Can you work these out from the drawing? Everything is in mm from the part's minimum corner. A direction names the side the tool comes from. Give positions to 0.01 mm unless a question says otherwise; leave off trailing zeros. Write each loop counter-clockwise with the first axis right and the second up, starting at its lowest first coordinate (ties: lowest second). Pieces come first, ordered by that corner, then holes. Notation, with made-up numbers: (80, 6.5) -> (136, 6.5) arc R17 ccw to (136, 33.5) -> close; hole circle Ø3 at (70.5, 86.5). An arc over 180 degrees is marked (long way). Return JSON: item names as keys, results as strings.
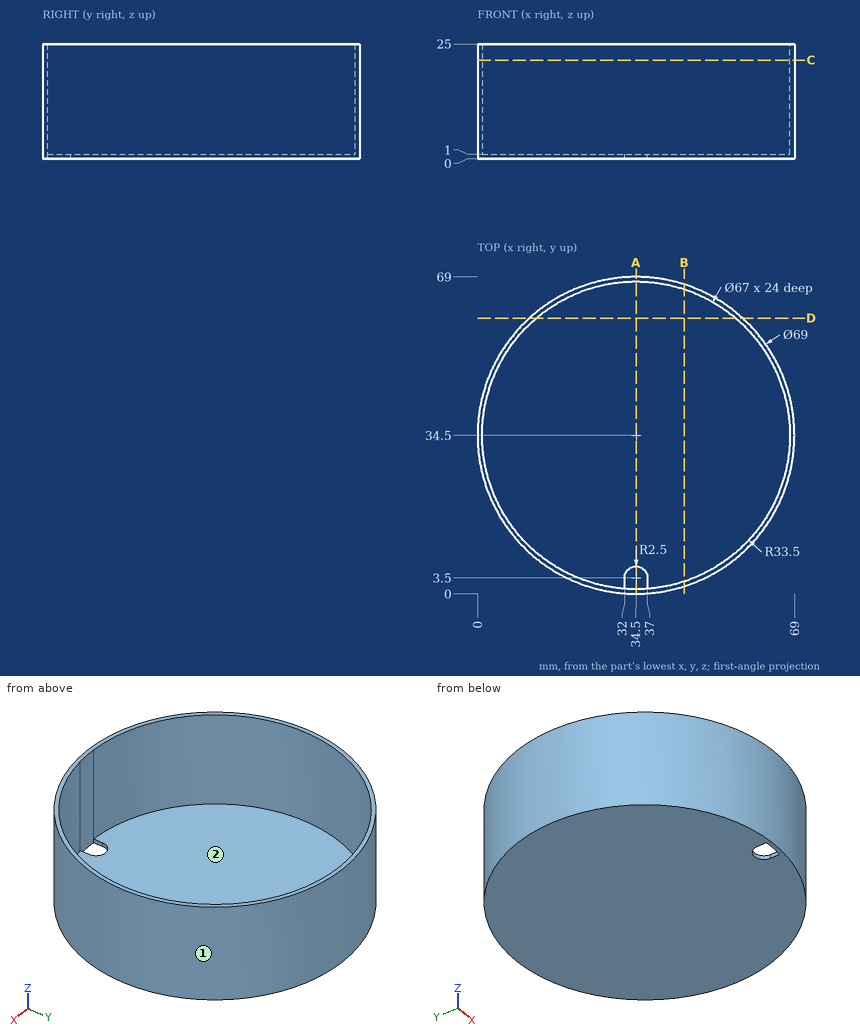
1. Suppose I cut it at B-B, the plane x = 45. List the corners of the cut face in (y, z) for me.
Taken from the geometry:
{"outline": "(1.64, 0) -> (67.36, 0) -> (67.36, 25) -> (66.31, 25) -> (66.31, 1) -> (2.69, 1) -> (2.69, 25) -> (1.64, 25) -> close"}
2. Suppose I cut it at D-D, the plane y = 60. List the corners of the cut face in (x, z) for me.
Taken from the geometry:
{"outline": "(11.26, 0) -> (57.74, 0) -> (57.74, 25) -> (56.23, 25) -> (56.23, 1) -> (12.77, 1) -> (12.77, 25) -> (11.26, 25) -> close"}
3. If I drill on line 1 (Y direction, x = 34.5, z = 6.5); line 2 (Z direction, x = 25, y = 46); line 3 (Y direction, x = 37, z = 22), over which ranges is the centre line in solid material (lowest first)? Write a range as [from, to].
Taken from the geometry:
{"line 1": "y = [0, 1], [68, 69]", "line 2": "z = [0, 1]", "line 3": "y = [0.09, 1.09], [67.91, 68.91]"}
4. Which directions (+Z, -Z, +X, -X, +Y, -Y) give clear straight access to the entire face, cutting with the end or side of a thin tool? Please do the marked faces 1 and 2.
Taken from the geometry:
{"face 1": "+Z, -Z", "face 2": "+Z"}
5. For pin 1 Ø1.1 at (y, z) = (3, 0.5) entering from -X; pin 2 Ø2 at (x, z) = (19, 14) entering from -Y (3 decimals); pin 3 Ø1.1 at (y, z) = (2, 0.5) entering from +X, each with a flat end and sliding along its axis, tell me the tip position at first contact or that it passes through.
Taken from the geometry:
{"pin 1": "stops at x = 19.26", "pin 2": "stops at y = 3.195", "pin 3": "stops at x = 47.52"}
6. Suppose I cut it at C-C, the plane z = 21.5. List the corners of the cut face in (x, y) for me, and give its area (3 significant figures).
Taken from the geometry:
{"outline": "circle Ø69 at (34.5, 34.5); hole (32, 1.09) arc R33.5 ccw to (37, 1.09) arc R33.5 ccw (long way) to start", "area": "214 mm²"}
7. Suppose I cut it at A-A, the plane x = 34.5. List the corners of the cut face in (y, z) for me.
Taken from the geometry:
{"outline": "(0, 0) -> (1, 0) -> (1, 25) -> (0, 25) -> close; (6, 0) -> (69, 0) -> (69, 25) -> (68, 25) -> (68, 1) -> (6, 1) -> close"}
